Verification items for the finished model (mm, model axes). Coordinates: 2 decimals unless noted, no trailing zeros. Write each loop counter-clockwise with the first axis right and the second up, starting at its lowest first coordinate (ties: lowest second). Pieces come first, ordered by that corner, then holes. Notation, with made-up numbers: M -25.5,32.25 L 11.5,32.25 A25 ccw 11.5,57.25 Z; hole C 87,84 d10. An arc over 180 degrees is marked long. One line per item, written item: value.
```python
from build123d import *

# Parameters (mm, degrees)
SKETCH_2_W          = 27
SKETCH_2_H          = 32
EXTRUDE_1_DEPTH     = 5
SKETCH_3_R          = 10
CUT_EXTRUDE_1_DEPTH = 64
SKETCH_5_R          = 1.6
CUT_EXTRUDE_2_DEPTH = 64


with BuildPart() as part:
    # 草图2 → 凸台-拉伸1 (new body)
    with BuildSketch(Plane.XY):
        with Locations((13.5, -16)):
            Rectangle(SKETCH_2_W, SKETCH_2_H)
    extrude(amount=EXTRUDE_1_DEPTH)

    # 草图3 → 切除-拉伸1 (cut)
    with BuildSketch(Plane.XY.offset(5)):
        with Locations((13.5, -16)):
            Circle(SKETCH_3_R)
    extrude(amount=-CUT_EXTRUDE_1_DEPTH, mode=Mode.SUBTRACT)

    # 草图5 → 切除-拉伸2 (cut)
    with BuildSketch(Plane.ZY):
        with Locations(Location((2.5, -3, 0), (0, 0, 270))):
            Circle(SKETCH_5_R)
        with Locations(Location((2.5, -29, 0), (0, 0, 270))):
            Circle(SKETCH_5_R)
    extrude(amount=-CUT_EXTRUDE_2_DEPTH, mode=Mode.SUBTRACT)


solid = part.part
```
Item 1: Go/stop test with a flat-tipped pin: P1, Ø12, axis at x = 13.5, y = -16, coming from the -Z side. Record where the tip stops, or that it passes through.
The answers:
P1: passes through
Item 2: Cross-section at B-B, the plane x = 13.5. Enter the section's corners in (y, z).
The answers:
outline: M -32,0 L -26,0 L -26,5 L -32,5 Z; M -6,0 L 0,0 L 0,5 L -6,5 Z; hole C -29,2.5 d3.2; hole C -3,2.5 d3.2
Item 3: Draft check along X on faces 1 (the face through (23.04, -13, 2.54)), 2 (the face through (13.31, -1.73, 1.53)), 3 (the face through (27, -16, 2)). Enter one of: released by +X, released by -X, zero draft, split by the parting line, or undercut.
The answers:
face 1: undercut
face 2: zero draft
face 3: released by +X
Item 4: Cross-section at A-A, the plane z = 2.5. Enter the section's corners in (x, y).
The answers:
outline: M 0,-32 L 27,-32 L 27,-30.6 L 0,-30.6 Z; M 0,-27.4 L 27,-27.4 L 27,-4.6 L 0,-4.6 Z; M 0,-1.4 L 27,-1.4 L 27,0 L 0,0 Z; hole C 13.5,-16 d20
Item 5: Cross-section at C-C, the plane y = -16. Enter the section's corners in (x, z).
The answers:
outline: M 0,0 L 3.5,0 L 3.5,5 L 0,5 Z; M 23.5,0 L 27,0 L 27,5 L 23.5,5 Z
Item 6: Scan lines: line 1 (Z direction, x = 20.25, y = -29); line 2 (Y direction, x = 2.25, z = 2.7); line 3 (Y direction, x = 13.5, z = 1.15). Record each from-to range of solid material in increasing order.
The answers:
line 1: z = 0 to 0.9, 4.1 to 5
line 2: y = -32 to -30.59, -27.41 to -4.59, -1.41 to 0
line 3: y = -32 to -29.86, -28.14 to -26, -6 to -3.86, -2.14 to 0
Item 7: Cross-section at D-D, the plane x = 2.25. Enter the section's corners in (y, z).
The answers:
outline: M -32,0 L 0,0 L 0,5 L -32,5 Z; hole C -29,2.5 d3.2; hole C -3,2.5 d3.2
